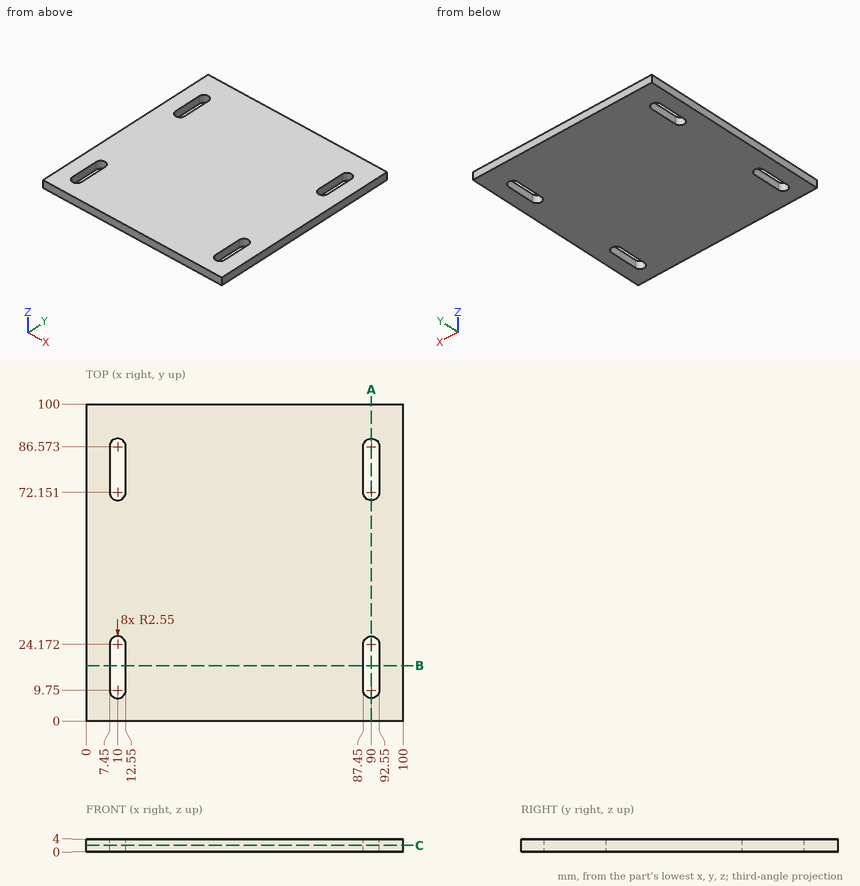
For this review, use the dimensioned drawing (mm, ordinates from the lowest corner) and the shaded views. Give positions to 0.01 mm unless a question says otherwise; leave off trailing zeros. Order: outer loops, then holes, each group sorted by start corner. A loop starts at its lowest first (then second) coordinate and runs counter-clockwise, first axis right, second up.
1. Add section B-B, the plane y = 17.5. State the section outline as (x, z) points, then the cut area to 3 significant figures.
Solution:
outline: (0, 0) - (7.45, 0) - (7.45, 4) - (0, 4) - close; (12.55, 0) - (87.45, 0) - (87.45, 4) - (12.55, 4) - close; (92.55, 0) - (100, 0) - (100, 4) - (92.55, 4) - close
area: 359 mm2
2. For pin 1 Ø1.2 at (y, z) = (81, 2.5) entering from -X, flat-tipped, find the tip position at first contact; note if it passes through.
Solution:
pin 1: stops at x = 0
3. To check wall thickness, follow L1, parallel to X at y = 83, z = 2.65. State the ranges of the line that lie inside material, in increasing order.
Solution:
L1: x = 0 to 7.45, 12.55 to 87.45, 92.55 to 100
4. Add section C-C, the plane z = 2. State the section outline as (x, y) points, then the cut area to 3 significant figures.
Solution:
outline: (0, 0) - (100, 0) - (100, 100) - (0, 100) - close; hole (7.45, 9.75) arc R2.55 ccw to (12.55, 9.75) - (12.55, 24.17) arc R2.55 ccw to (7.45, 24.17) - close; hole (7.45, 72.15) arc R2.55 ccw to (12.55, 72.15) - (12.55, 86.57) arc R2.55 ccw to (7.45, 86.57) - close; hole (87.45, 9.75) arc R2.55 ccw to (92.55, 9.75) - (92.55, 24.17) arc R2.55 ccw to (87.45, 24.17) - close; hole (87.45, 72.15) arc R2.55 ccw to (92.55, 72.15) - (92.55, 86.57) arc R2.55 ccw to (87.45, 86.57) - close
area: 9,620 mm2
5. Add section A-A, the plane x = 90. State the section outline as (y, z) points.
Solution:
outline: (0, 0) - (7.2, 0) - (7.2, 4) - (0, 4) - close; (26.72, 0) - (69.6, 0) - (69.6, 4) - (26.72, 4) - close; (89.12, 0) - (100, 0) - (100, 4) - (89.12, 4) - close
